Work out the finished part from the listing and answer in its coordinate system (mm). Face numbers are marked on the shaded views. A direction names the side the tool comes from. Round coordinates to 2 decimals unless told otherwise and drop trailing zeros. Order: outer loops, then holes, each group sorted by start corner. A loop starts at its lowest first (then second) coordinate and runs counter-clockwise, first axis right, second up. Notation, with made-up numbers: (32, 70.25) - (84, 70.25) arc R18 ccw to (84, 74.25) - close; hole circle Ø1 at (22, 46.25). An arc over 180 degrees is marked (long way). Put each result on its own line as item: value.
```python
from build123d import *
from build123d import SkipClean  # not in build123d's __all__

# Parameters (mm, degrees)
F1_DEPTH = 3.429
F0_R     = 1.397
F2_DEPTH = 3.048
F3_DEPTH = 2.032


with BuildPart() as f1:
    # F0 (on Top) → F1 (new body)
    with BuildSketch(Plane.XY):
        Polygon((15.24, -15.24), (15.24, 15.24), (-15.24, 15.24), (-15.24, -15.24), (-5.08, -15.24), (-5.08, -10.16), (5.08, -10.16), (5.08, -15.24), align=None)
        with BuildLine():
            ThreePointArc((3.2465476869, 2.227082647), (3.760427319, 1.1658281942), (3.937, 0))
            ThreePointArc((3.937, 0), (3.7477069339, -1.2060935857), (3.1980303594, -2.2962079219))
            ThreePointArc((3.1980303594, -2.2962079219), (5.1057127753, -2.3937225549), (6.0325, -4.064))
            ThreePointArc((6.0325, -4.064), (3.6195376595, -5.9816666754), (2.2962079219, -3.1980303594))
            ThreePointArc((2.2962079219, -3.1980303594), (0, -3.937), (-2.2962079219, -3.1980303594))
            ThreePointArc((-2.2962079219, -3.1980303594), (-2.1463333246, -3.6195376595), (-2.0955, -4.064))
            ThreePointArc((-2.0955, -4.064), (-5.7342774451, -5.1057127753), (-3.1980303594, -2.2962079219))
            ThreePointArc((-3.1980303594, -2.2962079219), (-3.937, 0), (-3.1980303594, 2.2962079219))
            ThreePointArc((-3.1980303594, 2.2962079219), (-5.7342774451, 5.1057127753), (-2.0955, 4.064))
            ThreePointArc((-2.0955, 4.064), (-2.1463333246, 3.6195376595), (-2.2962079219, 3.1980303594))
            ThreePointArc((-2.2962079219, 3.1980303594), (-0.0131703869, 3.9369779706), (2.2747600024, 3.2133216352))
            ThreePointArc((2.2747600024, 3.2133216352), (3.664202861, 5.9391021751), (6.0417570924, 4.0135718882))
            ThreePointArc((6.0417570924, 4.0135718882), (5.1333549146, 2.3549022836), (3.2465476869, 2.227082647))
        make_face(mode=Mode.SUBTRACT)
    extrude(amount=F1_DEPTH)

    # F0 (on Top) → F2 (join)
    with BuildSketch(Plane.XY):
        with BuildLine():
            ThreePointArc((-3.1980303594, 2.2962079219), (-2.7838793975, 2.7838793975), (-2.2962079219, 3.1980303594))
            ThreePointArc((-2.2962079219, 3.1980303594), (-2.1463333246, 3.6195376595), (-2.0955, 4.064))
            ThreePointArc((-2.0955, 4.064), (-5.7342774451, 5.1057127753), (-3.1980303594, 2.2962079219))
        make_face()
        with Locations((-4.064, 4.064)):
            Circle(F0_R, mode=Mode.SUBTRACT)
        with BuildLine():
            ThreePointArc((2.2747600024, 3.2133216352), (2.8043495655, 2.763257591), (3.2465476869, 2.227082647))
            ThreePointArc((3.2465476869, 2.227082647), (5.1333549146, 2.3549022836), (6.0417570924, 4.0135718882))
            ThreePointArc((6.0417570924, 4.0135718882), (3.664202861, 5.9391021751), (2.2747600024, 3.2133216352))
        make_face()
        with Locations((4.064, 4.064)):
            Circle(F0_R, mode=Mode.SUBTRACT)
        with BuildLine():
            ThreePointArc((-2.0955, -4.064), (-2.1463333246, -3.6195376595), (-2.2962079219, -3.1980303594))
            ThreePointArc((-2.2962079219, -3.1980303594), (-2.7838793975, -2.7838793975), (-3.1980303594, -2.2962079219))
            ThreePointArc((-3.1980303594, -2.2962079219), (-5.7342774451, -5.1057127753), (-2.0955, -4.064))
        make_face()
        with Locations((-4.064, -4.064)):
            Circle(F0_R, mode=Mode.SUBTRACT)
        with BuildLine():
            ThreePointArc((6.0325, -4.064), (5.1057127753, -2.3937225549), (3.1980303594, -2.2962079219))
            ThreePointArc((3.1980303594, -2.2962079219), (2.7838793975, -2.7838793975), (2.2962079219, -3.1980303594))
            ThreePointArc((2.2962079219, -3.1980303594), (3.6195376595, -5.9816666754), (6.0325, -4.064))
        make_face()
        with Locations((4.064, -4.064)):
            Circle(F0_R, mode=Mode.SUBTRACT)
    extrude(amount=F2_DEPTH)

    # F3 (cut): faces of the model
    f3_faces = [f1.faces().sort_by_distance(p)[0] for p in [
        (-2.8232493975, 2.8232493975, 3.048),
        (-5.4165696988, -5.4165696988, 3.048),
        (2.8440090574, 2.8023359547, 3.048),
        (5.4165696988, -5.4165696988, 3.048),
    ]]
    with SkipClean():  # cleaning this boolean's faces spoils the solid; the shape is the same uncleaned
        extrude(f3_faces, amount=-F3_DEPTH, mode=Mode.SUBTRACT)


solid = f1.part
```
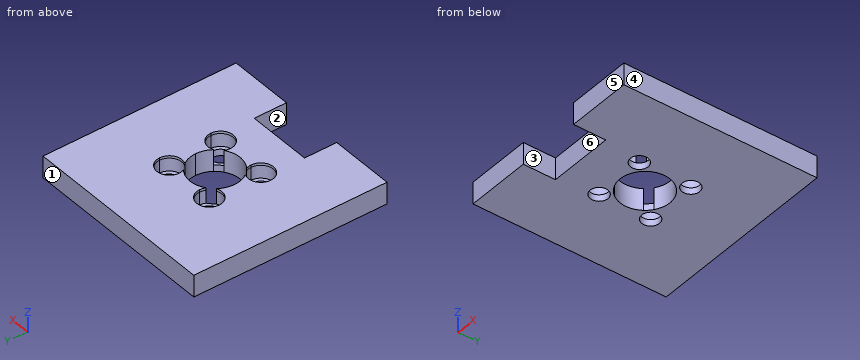
1) A cutting plane is placed at D-D on y = -12.5. Write down the section's boundary in (x, z).
Findings below:
outline: (-15.24, 0) - (-5.08, 0) - (-5.08, 3.43) - (-15.24, 3.43) - close; (5.08, 0) - (15.24, 0) - (15.24, 3.43) - (5.08, 3.43) - close
2) For a pull along X with two mould halves and no side action, classify the marked faces 3, 4, 5 and 6 as pulls with the +X half, pulls with the -X half, needs draft (parallel to the pull), parting line crosses it, or undercut.
Findings below:
face 3: undercut
face 4: pulls with the +X half
face 5: needs draft
face 6: undercut
3) Given pin 1 Ø2.5 at (x, y) = (-4.064, 4.064) entering from +Z; pin 2 Ø2 at (x, y) = (-4.5, -3.5) entering from +Z; pin 3 Ø1.7 at (x, z) = (-2.5, 2) entering from -Y, each flat-ended and moving along its own axis, determine where each tip first touches the part or whether it passes through.
Findings below:
pin 1: passes through
pin 2: stops at z = 1.02
pin 3: stops at y = -10.16
4) Straight lines are drawn through the part: L1, parallel to Y at x = -4, z = 0.2; L2, parallel to X at y = -11, z = 1.15; L3, parallel to X at y = -5, z = 2.95. For each, find the intervals that lie inside material, in ascending order. Write a range as from..to.
Findings below:
L1: y = -10.16..-5.46, -2.67..2.67, 5.46..15.24
L2: x = -15.24..-5.08, 5.08..15.24
L3: x = -15.24..-5.8, -2.33..2.33, 5.8..15.24
5) For the marked faces 1 and 2, determine the directions among +Z, -Z, +X, -X, +Y, -Y from which every point of the face is accessible in a straight line to the end or side of a thin tool.
Findings below:
face 1: +Z, -Z, +X, -X, +Y
face 2: +Z, -Z, -Y
6) A cutting plane is placed at C-C on x = -4.5. Write down the section's boundary in (y, z).
Findings below:
outline: (-10.16, 0) - (-5.39, 0) - (-5.39, 1.02) - (-5.98, 1.02) - (-5.98, 3.43) - (-10.16, 3.43) - close; (-2.74, 0) - (2.74, 0) - (2.74, 1.02) - (2.14, 1.02) - (2.14, 3.43) - (-2.14, 3.43) - (-2.14, 1.02) - (-2.74, 1.02) - close; (5.39, 0) - (15.24, 0) - (15.24, 3.43) - (5.98, 3.43) - (5.98, 1.02) - (5.39, 1.02) - close
7) A cutting plane is placed at A-A on z = 2.05. Write down the section's boundary in (x, y).
Findings below:
outline: (-15.24, -15.24) - (-5.08, -15.24) - (-5.08, -10.16) - (5.08, -10.16) - (5.08, -15.24) - (15.24, -15.24) - (15.24, 15.24) - (-15.24, 15.24) - close; hole (-3.2, -2.3) arc R1.97 ccw (long way) to (-2.3, -3.2) arc R3.94 ccw to (2.3, -3.2) arc R1.97 ccw (long way) to (3.2, -2.3) arc R3.94 ccw to (3.25, 2.23) arc R1.97 ccw (long way) to (2.27, 3.21) arc R3.94 ccw to (-2.3, 3.2) arc R1.97 ccw (long way) to (-3.2, 2.3) arc R3.94 ccw to start
8) A cutting plane is placed at B-B on y = 5. Write down the section's boundary in (x, z).
Findings below:
outline: (-15.24, 0) - (-5.1, 0) - (-5.1, 1.02) - (-5.8, 1.02) - (-5.8, 3.43) - (-15.24, 3.43) - close; (-3.03, 0) - (3.03, 0) - (3.03, 1.02) - (2.37, 1.02) - (2.37, 3.43) - (-2.33, 3.43) - (-2.33, 1.02) - (-3.03, 1.02) - close; (5.1, 0) - (15.24, 0) - (15.24, 3.43) - (5.78, 3.43) - (5.78, 1.02) - (5.1, 1.02) - close
